```python
from build123d import *

# Parameters (mm, degrees)
SKETCH1_W           = 19.812
SKETCH1_H           = 19.812
BOSS_EXTRUDE1_DEPTH = 19.812
SKETCH1_3_R         = 2.286
BOSS_EXTRUDE2_DEPTH = 6.35
CUT_EXTRUDE1_DEPTH  = 6.35
BOSS_EXTRUDE3_DEPTH = 6.35
SKETCH4_W           = 7.112
SKETCH4_H           = 7.112
BOSS_EXTRUDE4_DEPTH = 50.8


with BuildPart() as part:
    # Sketch1 → Boss-Extrude1 (new body)
    with BuildSketch(Plane(origin=(0, 0, 0), x_dir=(1, 0, 0), z_dir=(0, 1, 0))):
        with Locations((9.906, -9.906)):
            Rectangle(SKETCH1_W, SKETCH1_H)
    extrude(amount=BOSS_EXTRUDE1_DEPTH)

    # Sketch1_3 → Boss-Extrude2 (add)
    with BuildSketch(Plane(origin=(0, 0, 0), x_dir=(1, 0, 0), z_dir=(0, 1, 0))):
        Polygon((1.524, -6.858), (0, -6.858), (0, -12.954), (1.524, -12.954), (1.524, -14.732), (3.048, -14.732), (6.35, -12.954), (6.35, -6.858), (3.048, -5.08), (1.524, -5.08), align=None)
        Polygon((6.858, -18.288), (6.858, -19.812), (12.954, -19.812), (12.954, -18.288), (14.732, -18.288), (14.732, -16.764), (12.954, -13.462), (6.858, -13.462), (5.08, -16.764), (5.08, -18.288), align=None)
        Polygon((19.812, -12.954), (19.812, -6.858), (18.288, -6.858), (18.288, -5.08), (16.764, -5.08), (13.462, -6.858), (13.462, -12.954), (16.764, -14.732), (18.288, -14.732), (18.288, -12.954), align=None)
        with Locations(Location((9.906, -9.906, 0), (0, 0, 270))):
            Circle(SKETCH1_3_R)
    extrude(amount=-BOSS_EXTRUDE2_DEPTH)

    # Sketch1_5 → Cut-Extrude1 (cut)
    with BuildSketch(Plane(origin=(0, 0, 0), x_dir=(1, 0, 0), z_dir=(0, 1, 0))):
        Polygon((12.954, 0), (12.954, -1.524), (14.732, -1.524), (14.732, -3.048), (12.954, -6.35), (6.858, -6.35), (5.08, -3.048), (5.08, -1.524), (6.858, -1.524), (6.858, 0), align=None)
    extrude(amount=CUT_EXTRUDE1_DEPTH, mode=Mode.SUBTRACT)

    # Sketch3 → Boss-Extrude3 (add)
    with BuildSketch(Plane(origin=(0, 0, 0), x_dir=(-1, 0, 0), z_dir=(0, 0, -1))):
        Polygon((-13.462, 9.906), (-19.812, 9.906), (-19.812, 6.858), (-18.288, 6.858), (-18.288, 5.08), (-16.764, 5.08), (-13.462, 6.858), align=None)
        Polygon((-19.812, 12.954), (-19.812, 9.906), (-13.462, 9.906), (-13.462, 12.954), (-16.764, 14.732), (-18.288, 14.732), (-18.288, 12.954), align=None)
        Polygon((-6.858, 19.812), (-12.954, 19.812), (-12.954, 18.288), (-14.732, 18.288), (-14.732, 16.764), (-12.954, 13.462), (-9.906, 13.462), (-6.858, 13.462), (-5.08, 16.764), (-5.08, 18.288), (-6.858, 18.288), align=None)
        with BuildLine():
            ThreePointArc((-9.906, 12.192), (-11.522446102, 11.522446102), (-12.192, 9.906))
            Line((-12.192, 9.906), (-7.62, 9.906))
            ThreePointArc((-7.62, 9.906), (-8.289553898, 11.522446102), (-9.906, 12.192))
        make_face()
        with BuildLine():
            Line((-7.62, 9.906), (-12.192, 9.906))
            ThreePointArc((-12.192, 9.906), (-9.906, 7.62), (-7.62, 9.906))
        make_face()
        Polygon((0, 9.906), (-6.35, 9.906), (-6.35, 6.858), (-3.048, 5.08), (-1.524, 5.08), (-1.524, 6.858), (0, 6.858), align=None)
        Polygon((-6.35, 12.954), (-6.35, 9.906), (0, 9.906), (0, 12.954), (-1.524, 12.954), (-1.524, 14.732), (-3.048, 14.732), align=None)
    extrude(amount=BOSS_EXTRUDE3_DEPTH)

    # Sketch4 → Boss-Extrude4 (add)
    with BuildSketch(Plane.ZY):
        with Locations((3.556, 16.256)):
            Rectangle(SKETCH4_W, SKETCH4_H)
        with Locations((16.256, 16.256)):
            Rectangle(SKETCH4_W, SKETCH4_H)
        with Locations((16.256, 3.556)):
            Rectangle(SKETCH4_W, SKETCH4_H)
        with Locations((3.556, 3.556)):
            Rectangle(SKETCH4_W, SKETCH4_H)
    extrude(amount=BOSS_EXTRUDE4_DEPTH)


solid = part.part
```
Can you work these out from the model? Positions are in its coordinate system, mm. A direction names the side the tool comes from. Give positions to 0.01 mm unless a question says otherwise; leave off trailing zeros. Order: outer loops, then holes, each group sorted by start corner. A loop starts at its lowest first (then second) coordinate and runs counter-clockwise, first axis right, second up. Notation, with made-up numbers: (33.25, 18.25) - (70.25, 18.25) arc R21 cw to (70.25, 33.25) - close; hole circle Ø8 at (31, 63.25). An arc over 180 degrees is marked (long way). Use a Markdown table: item, result. Add a question column.
Q1. If we mould it in two halves opening along Y, with no side actions, what happens to faces 1 (the flat face through (3, -6.35, 10)), 2 (the flat face through (19, 12.954, -3)), 3 (the flat face through (-25, 12.7, 4))? For each: released by +Y, released by -Y, zero draft, split by the parting line, or undercut.
Q2. If we section it at C-C on x = -2: Write out the boundary of the cut face in (y, z), plus the area to 3 significant figures.
Q3. On a 3-axis mill with a long thin cutter (end or side, diameter ignored), from which of +Z, -Z, +X, -X, +Y, -Y can I reach the whole of each face in a straight line? I mean faces 4 (the flat face through (5.08, 3, 2)), 5 (the flat face through (-25, 4, 12.7)), 6 (the flat face through (4.72, 5.98, -3.13)), 7 (the flat face through (12.954, -3, 19)). Say none if no direction works.
Q4. Please list where these lines run through material, in increasing order: line 1 along Z through (x, y) = (-39, 15.25); line 2 along X through (y, z) = (4, 12).
Q5. I'm going to push flat-ended pins straight in: pin 1 (8 mm diameter, centred on x = -38, z = 4, fed in from -Y); pin 2 (0.9 mm diameter, centred on y = 14, z = -3.5, fed in from -X); pin 3 (1.2 mm diameter, centred on x = 0.5, z = -3, fed in from +Y). Where does each tip first touch, or does it pass through?
Q6. If we section it at D-D on y = 2: Write out the boundary of the cut face in (x, z).
Q7. If we section it at A-A on y = -4: Count the separate pieces of the cut face and the enclosed holes in it, plus the area to 3 significant figures.
Answers follow:
| question | item | result |
|---|---|---|
| 1 | face 1 | released by -Y |
| 1 | face 2 | released by +Y |
| 1 | face 3 | undercut |
| 2 | outline | (0, 0) - (7.11, 0) - (7.11, 7.11) - (0, 7.11) - close; (0, 12.7) - (7.11, 12.7) - (7.11, 19.81) - (0, 19.81) - close; (12.7, 0) - (19.81, 0) - (19.81, 7.11) - (12.7, 7.11) - close; (12.7, 12.7) - (19.81, 12.7) - (19.81, 19.81) - (12.7, 19.81) - close |
| 2 | area | 202 mm^2 |
| 3 | face 4 | -Y |
| 3 | face 5 | -X, +Y, -Y |
| 3 | face 6 | -Z, -Y |
| 3 | face 7 | +Z, +X, -Y |
| 4 | line 1 | z = 0 to 7.11, 12.7 to 19.81 |
| 4 | line 2 | x = 0 to 19.81 |
| 5 | pin 1 | stops at y = 0 |
| 5 | pin 2 | stops at x = 1.52 |
| 5 | pin 3 | stops at y = 12.95 |
| 6 | outline | (-50.8, 0) - (6.86, 0) - (6.86, 1.52) - (5.08, 1.52) - (5.08, 3.05) - (6.86, 6.35) - (12.95, 6.35) - (14.73, 3.05) - (14.73, 1.52) - (12.95, 1.52) - (12.95, 0) - (19.81, 0) - (19.81, 19.81) - (-50.8, 19.81) - (-50.8, 12.7) - (0, 12.7) - (0, 7.11) - (-50.8, 7.11) - close |
| 7 | separate pieces | 4 |
| 7 | enclosed holes | 0 |
| 7 | area | 166 mm^2 |
